Here's how the part is built. I have some questions about the finished solid (model axes, mm). Face numbers are marked on the shaded views. Round coordinates to 2 decimals unless told otherwise and drop trailing zeros. Order: outer loops, then holes, each group sorted by start corner. A loop starts at its lowest first (then second) coordinate and runs counter-clockwise, first axis right, second up. Notation, with made-up numbers: M -3.5,-26.75 L 35.5,-26.75 A12 cw 35.5,-7.75 Z; hole C 3,11.5 d7. An arc over 180 degrees is marked long. Write each question's results on one line, items separated by ' | '. Start each with the question number.
```python
from build123d import *

# Parameters (mm, degrees)
ESQUISSE1_W                                  = 270
ESQUISSE1_H                                  = 270
EXTRUSION1_DEPTH                             = 15
CONG_2_R                                     = 4
EXTRUSION2_DEPTH                             = 13
CONG_3_R                                     = 4
CHAMBRAGE_POUR_VIS_T_TE_RONDE_BOMB_E_A_COUNT = 2
CHAMBRAGE_POUR_VIS_T_TE_RONDE_BOMB_E_A_PITCH = 258
CHAMBRAGE_POUR_VIS_T_TE_RONDE_BOMB_2_COUNT   = 2
CHAMBRAGE_POUR_VIS_T_TE_RONDE_BOMB_2_PITCH   = 364.867099092
CHAMBRAGE_POUR_VIS_T_TE_RONDE_BOMB_3_COUNT   = 2
CHAMBRAGE_POUR_VIS_T_TE_RONDE_BOMB_3_PITCH   = 258


with BuildPart() as part:
    # Esquisse1 → Extrusion1 (new body)
    with BuildSketch(Plane.XY):
        with Locations((135, -135)):
            Rectangle(ESQUISSE1_W, ESQUISSE1_H)
    extrude(amount=EXTRUSION1_DEPTH)

    # Congé2
    cong_2_edges = [part.edges().sort_by_distance(p)[0] for p in [
        (0, 0, 7.5),
        (270, 0, 7.5),
        (270, -270, 7.5),
        (0, -270, 7.5),
    ]]
    fillet(cong_2_edges, radius=CONG_2_R)

    # Esquisse2 → Extrusion2 (cut)
    with BuildSketch(Plane.XY.offset(15)):
        Polygon((12, -2), (12, -19), (2, -19), (2, -251), (12, -251), (12, -268), (258, -268), (258, -251), (268, -251), (268, -19), (258, -19), (258, -2), align=None)
    extrude(amount=-EXTRUSION2_DEPTH, mode=Mode.SUBTRACT)

    # Congé3
    cong_3_edges = [part.edges().sort_by_distance(p)[0] for p in [
        (258, -19, 8.5),
        (258, -251, 8.5),
        (12, -251, 8.5),
        (12, -19, 8.5),
    ]]
    fillet(cong_3_edges, radius=CONG_3_R)

    # Esquisse6 → Chambrage pour vis à tête ronde bombée #41 (revolve, cut)
    with BuildSketch(Plane(origin=(264, -6, 0), x_dir=(0, 1, 0), z_dir=(1, 0, 0))):
        Polygon((0, 0), (0, 15), (1.63195, 15), (1.63195, 4.031996), (3.175, 4.031996), (3.175, 0.635), (3.81, 0), align=None)
    chambrage_pour_vis_t_te_ronde_bomb_e = revolve(axis=Axis((264, -6, -6.35), (0, 0, 1)), mode=Mode.SUBTRACT)

    # Chambrage pour vis à tête ronde bombée #41 a: Chambrage pour vis à tête ronde bombée #41 ×2
    with Locations(*[(-i * CHAMBRAGE_POUR_VIS_T_TE_RONDE_BOMB_E_A_PITCH, 0, 0) for i in range(1, CHAMBRAGE_POUR_VIS_T_TE_RONDE_BOMB_E_A_COUNT)]):
        add(chambrage_pour_vis_t_te_ronde_bomb_e, mode=Mode.SUBTRACT)

    # Chambrage pour vis _ t_te ronde bomb 2: Chambrage pour vis à tête ronde bombée #41 ×2
    with Locations(*[Vector(-0.707106781, -0.707106781, 0) * (i * CHAMBRAGE_POUR_VIS_T_TE_RONDE_BOMB_2_PITCH) for i in range(1, CHAMBRAGE_POUR_VIS_T_TE_RONDE_BOMB_2_COUNT)]):
        add(chambrage_pour_vis_t_te_ronde_bomb_e, mode=Mode.SUBTRACT)

    # Chambrage pour vis _ t_te ronde bomb 3: Chambrage pour vis à tête ronde bombée #41 ×2
    with Locations(*[(0, -i * CHAMBRAGE_POUR_VIS_T_TE_RONDE_BOMB_3_PITCH, 0) for i in range(1, CHAMBRAGE_POUR_VIS_T_TE_RONDE_BOMB_3_COUNT)]):
        add(chambrage_pour_vis_t_te_ronde_bomb_e, mode=Mode.SUBTRACT)


solid = part.part
```
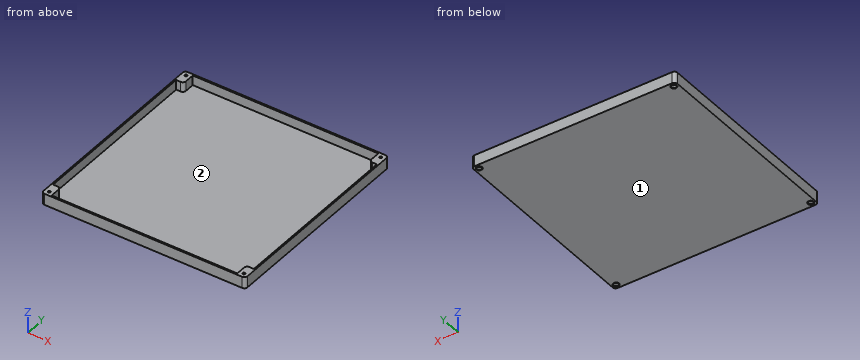
(1) If we mould it in two halves opening along X, with no side actions, what happens to the marked faces 1 and 2? For each: pulls with the +X half, pulls with the -X half, needs draft (parallel to the pull), parting line crosses it, or undercut.
(2) I want a section at A-A on x = 199. Write out the boundary of the cut face in (y, z).
(3) Please list where these lines run through material, in increasing order: line 1 (Y direction, x = 264, z = 2.3) (3 decimals); line 2 (X direction, y = -264, z = 3.05) (3 decimals); line 3 (Y direction, x = 13.5, z = 6.75).
(4) I want a section at C-C on z = 7.75. Write out the boundary of the cut face in (x, y), and give its area (3 significant figures).
(5) I want a section at B-B on y = -94. Write out the boundary of the cut face in (x, z), and give its area (3 significant figures).
(6) I'm going to push flat-ended pins straight in: pin 1 Ø2.5 at (x, y) = (264, -264) entering from +Z; pin 2 Ø3 at (x, y) = (263, -262.5) entering from -Z. Where does each tip first touch, or does it pass through?
Solutions:
1) face 1: needs draft | face 2: undercut
2) outline: M -270,0 L 0,0 L 0,15 L -2,15 L -2,2 L -268,2 L -268,15 L -270,15 Z
3) line 1: -270 to -267.175, -260.825 to -251, -19 to -9.175, -2.825 to 0 | line 2: 0 to 2.825, 9.175 to 12, 258 to 260.825, 267.175 to 270 | line 3: -270 to -268, -2 to 0
4) outline: M 0,-266 A4 ccw 4,-270 L 266,-270 A4 ccw 270,-266 L 270,-4 A4 ccw 266,0 L 4,0 A4 ccw 0,-4 Z; hole M 2,-251 L 8,-251 A4 cw 12,-255 L 12,-268 L 258,-268 L 258,-255 A4 cw 262,-251 L 268,-251 L 268,-19 L 262,-19 A4 cw 258,-15 L 258,-2 L 12,-2 L 12,-15 A4 cw 8,-19 L 2,-19 Z; hole C 6,-264 d3.26; hole C 6,-6 d3.26; hole C 264,-264 d3.26; hole C 264,-6 d3.26 | area: 2,760 mm^2
5) outline: M 0,0 L 270,0 L 270,15 L 268,15 L 268,2 L 2,2 L 2,15 L 0,15 Z | area: 592 mm^2
6) pin 1: through | pin 2: z = 0.51
